Autodesk Inventor part; units mm, degrees
ref_plane "YZ Plane" through (0, 0, 0) normal (1, 0, 0) x (0, 1, 0)
ref_plane "XZ Plane" through (0, 0, 0) normal (0, 1, 0) x (-1, 0, 0)
ref_plane "XY Plane" through (0, 0, 0) normal (0, 0, 1) x (1, 0, 0)
sketch "Sketch1" plane through (0, 0, 0) normal (0, 0, 1) x (1, 0, 0)
  line L0 (45, -50) -> (-45, -50)
  line L1 (-45, -50) -> (-45, 50)
  line L2 (-45, 50) -> (45, 50)
  line L3 (45, 50) -> (45, -50)
  line L4 (45, -50) -> (-45, 50) construction
  line L5 (-45, -50) -> (45, 50) construction
  line L6 (53, 58) -> (-53, 58)
  line L7 (-53, 58) -> (-53, 54.5)
  line L8 (-53, -58) -> (53, -58)
  line L9 (53, -58) -> (53, -54.5)
  line L10 (-20, 50) -> (20, 50)
  line L11 (20, 50) -> (20, 54)
  line L12 (20, 54) -> (-20, 54)
  line L13 (-20, 54) -> (-20, 50)
  line L14 (-20, -50) -> (20, -50)
  line L15 (20, -50) -> (20, -54)
  line L16 (20, -54) -> (-20, -54)
  line L17 (-20, -54) -> (-20, -50)
  line L18 (-45, 20) -> (-49, 20)
  line L19 (-49, 20) -> (-49, -20)
  line L20 (-49, -20) -> (-45, -20)
  line L21 (-45, -20) -> (-45, 20)
  line L22 (45, 20) -> (49, 20)
  line L23 (49, 20) -> (49, -20)
  line L24 (49, -20) -> (45, -20)
  line L25 (45, -20) -> (45, 20)
  line L26 (-53, 6.5) -> (-77, 6.5)
  line L27 (-100, 6.5) -> (-100, -6.5)
  line L28 (-100, -6.5) -> (-92, -6.5)
  line L29 (-53, -6.5) -> (-53, 6.5) construction
  line L30 (-53, 0) -> (53, 0)
  circle A0 centre (-92, 0) radius 1.45
  circle A1 centre (-77, 0) radius 1.45
  line L31 (0, 50) -> (0, -50)
  line L32 (-53, 6.5) -> (-53, -6.5) construction
  line L33 (-53, -6.5) -> (-53, -44.5)
  line L34 (53, 6.5) -> (53, 44.5)
  line L35 (53, -6.5) -> (53, 6.5) construction
  line L36 (-92, -6.5) -> (-77, -6.5) construction
  line L37 (-77, -6.5) -> (-77, -44.5)
  line L38 (-77, -58) -> (-92, -58) construction
  line L39 (-92, -58) -> (-92, -54.5) construction
  line L40 (-92, -58) -> (-77, -58) construction
  line L41 (-77, -58) -> (-77, -58.5) construction
  line L42 (-77, -58.5) -> (-81.5, -58.5) construction
  line L43 (-92, -58.5) -> (-92, -58) construction
  line L44 (-92, -54.5) -> (-87.5, -54.5)
  line L45 (-87.5, -54.5) -> (-87.5, -58.5)
  line L46 (-81.5, -58.5) -> (-81.5, -54.5)
  line L47 (-81.5, -54.5) -> (-77, -54.5)
  line L48 (-77, 6.5) -> (-77, 44.5)
  line L49 (-77, 58) -> (-92, 58) construction
  line L50 (-92, 58) -> (-92, 54.5) construction
  line L51 (-92, 58) -> (-77, 58) construction
  line L52 (-77, 58) -> (-77, 58.5) construction
  line L53 (-77, 58.5) -> (-81.5, 58.5) construction
  line L54 (-92, 58.5) -> (-92, 58) construction
  line L55 (-92, 54.5) -> (-87.5, 54.5)
  line L56 (-87.5, 54.5) -> (-87.5, 58.5)
  line L57 (-81.5, 58.5) -> (-81.5, 54.5)
  line L58 (-81.5, 54.5) -> (-77, 54.5)
  line L59 (-77, 6.5) -> (-92, 6.5) construction
  line L60 (-92, 6.5) -> (-100, 6.5)
  line L61 (-92, -6.5) -> (-77, -6.5) construction
  line L62 (-77, -6.5) -> (-53, -6.5)
  line L63 (-77, 54.5) -> (-77, 58) construction
  line L64 (-92, 54.5) -> (-92, 6.5)
  line L65 (-87.5, 58.5) -> (-92, 58.5) construction
  line L66 (-81.5, 58.5) -> (-87.5, 58.5)
  line L67 (-92, -54.5) -> (-92, -6.5)
  line L68 (-87.5, -58.5) -> (-92, -58.5) construction
  line L69 (-81.5, -58.5) -> (-87.5, -58.5)
  line L70 (-77, -54.5) -> (-77, -58) construction
  line L71 (-77, 54.5) -> (-71.5, 54.5)
  line L72 (-53, 54.5) -> (-53, 44.5) construction
  line L73 (-53, 44.5) -> (-77, 44.5)
  line L74 (-77, 44.5) -> (-77, 54.5) construction
  line L75 (-77, -54.5) -> (-71.5, -54.5)
  line L76 (-53, -54.5) -> (-53, -54)
  line L77 (-53, -44.5) -> (-77, -44.5)
  line L78 (-77, -44.5) -> (-77, -54.5) construction
  line L79 (-71.5, 54.5) -> (-65.5, 54.5) construction
  line L80 (-65.5, 54.5) -> (-65.5, 58.5)
  line L81 (-65.5, 58.5) -> (-71.5, 58.5)
  line L82 (-71.5, 58.5) -> (-71.5, 54.5)
  line L83 (-71.5, -54.5) -> (-65.5, -54.5) construction
  line L84 (-65.5, -54.5) -> (-65.5, -58.5)
  line L85 (-65.5, -58.5) -> (-71.5, -58.5)
  line L86 (-71.5, -58.5) -> (-71.5, -54.5)
  line L87 (-71.5, 54.5) -> (-65.5, 54.5) construction
  line L88 (-65.5, 54.5) -> (-53, 54.5)
  line L89 (-77, 44.5) -> (-77, 54.5) construction
  line L90 (-53, 44.5) -> (-53, 6.5)
  line L91 (-53, 54.5) -> (-53, 44.5) construction
  line L92 (-77, -44.5) -> (-77, -54.5) construction
  line L93 (-53, -44.5) -> (-53, -54.5) construction
  line L94 (-53, -54) -> (-53, -44.5) construction
  line L95 (-65.5, -54.5) -> (-53, -54.5)
  line L96 (-71.5, -54.5) -> (-65.5, -54.5) construction
  line L97 (-53, -54.5) -> (-53, -58)
  line L98 (53, 6.5) -> (77, 6.5)
  line L99 (100, 6.5) -> (100, -6.5)
  line L100 (100, -6.5) -> (92, -6.5)
  circle A2 centre (92, 0) radius 1.45
  circle A3 centre (77, 0) radius 1.45
  line L101 (92, -6.5) -> (77, -6.5) construction
  line L102 (77, -6.5) -> (77, -44.5)
  line L103 (77, -58) -> (92, -58) construction
  line L104 (92, -58) -> (92, -54.5) construction
  line L105 (92, -58) -> (77, -58) construction
  line L106 (77, -58) -> (77, -58.5) construction
  line L107 (77, -58.5) -> (81.5, -58.5) construction
  line L108 (92, -58.5) -> (92, -58) construction
  line L109 (92, -54.5) -> (87.5, -54.5)
  line L110 (87.5, -54.5) -> (87.5, -58.5)
  line L111 (81.5, -58.5) -> (81.5, -54.5)
  line L112 (81.5, -54.5) -> (77, -54.5)
  line L113 (92, 54.5) -> (87.5, 54.5)
  line L114 (92, 58) -> (92, 54.5) construction
  line L115 (77, 6.5) -> (77, 44.5)
  line L116 (81.5, 54.5) -> (77, 54.5)
  line L117 (77, 58) -> (92, 58) construction
  line L118 (92, 58) -> (77, 58) construction
  line L119 (77, 58) -> (77, 58.5) construction
  line L120 (77, 58.5) -> (81.5, 58.5) construction
  line L121 (81.5, 58.5) -> (81.5, 54.5)
  line L122 (92, 58.5) -> (92, 58) construction
  line L123 (87.5, 54.5) -> (87.5, 58.5)
  line L124 (77, 6.5) -> (92, 6.5) construction
  line L125 (92, 6.5) -> (100, 6.5)
  line L126 (92, -6.5) -> (77, -6.5) construction
  line L127 (77, -6.5) -> (53, -6.5)
  line L128 (77, 54.5) -> (77, 58) construction
  line L129 (92, 54.5) -> (92, 6.5)
  line L130 (87.5, 58.5) -> (92, 58.5) construction
  line L131 (81.5, 58.5) -> (87.5, 58.5)
  line L132 (92, -54.5) -> (92, -6.5)
  line L133 (87.5, -58.5) -> (92, -58.5) construction
  line L134 (81.5, -58.5) -> (87.5, -58.5)
  line L135 (77, -54.5) -> (77, -58) construction
  line L136 (77, 54.5) -> (71.5, 54.5)
  line L137 (53, 44.5) -> (77, 44.5)
  line L138 (77, 44.5) -> (77, 54.5) construction
  line L139 (77, -54.5) -> (71.5, -54.5)
  line L140 (53, -44.5) -> (77, -44.5)
  line L141 (77, -44.5) -> (77, -54.5) construction
  line L142 (71.5, 54.5) -> (65.5, 54.5) construction
  line L143 (65.5, 54.5) -> (65.5, 58.5)
  line L144 (65.5, 58.5) -> (71.5, 58.5)
  line L145 (71.5, 58.5) -> (71.5, 54.5)
  line L146 (71.5, -54.5) -> (65.5, -54.5) construction
  line L147 (65.5, -54.5) -> (65.5, -58.5)
  line L148 (65.5, -58.5) -> (71.5, -58.5)
  line L149 (71.5, -58.5) -> (71.5, -54.5)
  line L150 (71.5, 54.5) -> (65.5, 54.5) construction
  line L151 (65.5, 54.5) -> (53, 54.5)
  line L152 (77, 44.5) -> (77, 54.5) construction
  line L153 (77, -44.5) -> (77, -54.5) construction
  line L154 (65.5, -54.5) -> (53, -54.5)
  line L155 (71.5, -54.5) -> (65.5, -54.5) construction
  line L156 (53, 44.5) -> (53, 54.5) construction
  line L157 (53, 54.5) -> (53, 58)
  line L158 (53, -44.5) -> (53, -6.5)
  line L159 (53, -54.5) -> (53, -44.5) construction
  point P0 (0, 0)
  point P1 (0, 54)
  point P2 (0, 0)
  point P3 (-49, 0)
  point P4 (0, 0)
  point P5 (-53, 0)
  point P6 (0, 0)
  point P7 (0, 0)
  point P8 (-84.5, -58)
  point P9 (-84.5, 58)
  point P10 (-65, 44.5)
  point P11 (-81.5, 56.5)
  point P12 (-71.5, 56.5)
  point P13 (84.5, -58)
  point P14 (84.5, 58)
  point P15 (65, 44.5)
  point P16 (81.5, 56.5)
  point P17 (71.5, 56.5)
  dimension "d0" = 100
  dimension "d1" = 90
  dimension "d2" = 8
  dimension "d3" = 4
  dimension "d4" = 4
  dimension "d5" = 40
  dimension "d6" = 40
  dimension "d7" = 4
  dimension "d8" = 4
  dimension "d9" = 13
  dimension "d10" = 47
  dimension "d11" = 2.9
  dimension "d12" = 15
  dimension "d13" = 24
  dimension "d14" = 4
  dimension "d15" = 4
  dimension "d16" = 15
  dimension "d17" = 0.5
  dimension "d18" = 6
  dimension "d19" = 4.5
  dimension "d20" = 4.5
  dimension "d21" = 4
  dimension "d24" = 10
  dimension "d25" = 10
  dimension "d27" = 10
  dimension "d28" = 6
extrude "Extrusion1" add sketch "Sketch1" along normal blind 4
properties part number "DoorFrameRear_V2" material "Wood (Oak)"
Model file for the job. Use its own axes, mm. A direction names the side the tool comes from. Give positions to 0.01 mm unless a question says otherwise; leave off trailing zeros. Order: outer loops, then holes, each group sorted by start corner. A loop starts at its lowest first (then second) coordinate and runs counter-clockwise, first axis right, second up. Notation, with made-up numbers: (61, -12.5) - (70, -12.5) arc R28 cw to (70, 20.5) - close; hole circle Ø5 at (-0.5, -6). An arc over 180 degrees is marked (long way). Return JSON: item names as keys, results as strings.
1) 3-axis set-ups, long thin cutter, end or side, ignore diameter. For faces 1 (the flat face through (-45, 35, 2)), 2 (the flat face through (87.5, 56, 2)), 3 (the flat face through (-81.5, 57, 2)): which of +Z, -Z, +X, -X, +Y, -Y reach the whole face in a straight line?
Geometry says:
{"face 1": "+Z, -Z", "face 2": "+Z, -Z, +X, +Y", "face 3": "+Z, -Z, +Y"}
2) Flat gauge pins, fed straight in: P1, Ø1.2, axis at x = 89.5, z = 1.5, coming from the +Y side; P2, Ø2, axis at y = -56.5, z = 3, coming from the -X side; P3, Ø6, axis at x = -39, y = -45, coming from the +Z side; P4, Ø1.2, axis at x = 56.5, z = 1.5, coming from the -Y side. Where does each tip first touch, or does it go through?
Geometry says:
{"P1": "y = 54.5", "P2": "x = -87.5", "P3": "through", "P4": "y = -54.5"}
3) Pull direction X, two halves, no side cores. Call faces 4 (the flat face through (92, -31, 2)), 5 (the flat face through (-53, -25, 2)), 6 (the flat face through (-68, 58.5, 2)): pulls with the +X half, pulls with the -X half, needs draft (parallel to the pull), parting line crosses it, or undercut.
Geometry says:
{"face 4": "pulls with the +X half", "face 5": "undercut", "face 6": "needs draft"}
4) Cut at B-B, the plane x = 59.5. Give the cut face in (y, z), plus the area to 3 significant figures.
Geometry says:
{"outline": "(-54.5, 0) - (-44.5, 0) - (-44.5, 4) - (-54.5, 4) - close; (-6.5, 0) - (6.5, 0) - (6.5, 4) - (-6.5, 4) - close; (44.5, 0) - (54.5, 0) - (54.5, 4) - (44.5, 4) - close", "area": "132 mm²"}
5) Cut at A-A, the plane y = -27. Give the cut face in (x, z).
Geometry says:
{"outline": "(-92, 0) - (-77, 0) - (-77, 4) - (-92, 4) - close; (-53, 0) - (-45, 0) - (-45, 4) - (-53, 4) - close; (45, 0) - (53, 0) - (53, 4) - (45, 4) - close; (77, 0) - (92, 0) - (92, 4) - (77, 4) - close"}
6) Cut at C-C, the plane y = -3.5. Give the cut face in (x, z), plus the area to 3 significant figures.
Geometry says:
{"outline": "(-100, 0) - (-49, 0) - (-49, 4) - (-100, 4) - close; (49, 0) - (100, 0) - (100, 4) - (49, 4) - close", "area": "408 mm²"}
7) Probe line 1 (Y direction, x = 67, z = 2.6); line 2 (X direction, y = -27, z = 3.5); line 3 (X direction, y = -15.5, z = 1.5). List the from-to ranges inside material, lowest first. Write a range as from..to.
Geometry says:
{"line 1": "-58.5..-44.5, -6.5..6.5, 44.5..58.5", "line 2": "-92..-77, -53..-45, 45..53, 77..92", "line 3": "-92..-77, -53..-49, 49..53, 77..92"}
8) Cut at D-D, the plane x = 9. Give the cut face in (y, z), plus the area to 3 significant figures.
Geometry says:
{"outline": "(-58, 0) - (-54, 0) - (-54, 4) - (-58, 4) - close; (54, 0) - (58, 0) - (58, 4) - (54, 4) - close", "area": "32.0 mm²"}
